```python
from build123d import *

# Parameters (mm, degrees)
F0_W     = 27.4
F0_H     = 2.1
F1_DEPTH = 5
F2_DEPTH = 4
F3_D     = 5
F4_R     = 4.9999


# Not quite as in the source:
# - a fillet or chamfer is up to 0.001 mm smaller than in the source, because OpenCascade refuses the exact size
# - ends of sketch curves that miss each other by under 0.0002 mm in the source are joined
# - a feature names something its author has since deleted; it is built from what else it names


with BuildPart() as f1:
    # F0 (on Top) → F1 (new body)
    with BuildSketch(Plane.XY):
        with BuildLine():
            Line((-35, 2.1762e-06), (-35, -40))
            Line((-35, -40), (-27, -40))
            Line((-27, -40), (-27, -22.2710574513))
            ThreePointArc((-27, -22.2710574513), (-32.9393385518, -11.8321585422), (-35, 2.1762e-06))
        make_face()
        with BuildLine():
            Line((-27, -22.2710574513), (-27, -40))
            Line((-27, -40), (27, -40))
            Line((27, -40), (27, -22.2710574513))
            ThreePointArc((27, -22.2710574513), (0, -35), (-27, -22.2710574513))
        make_face()
        with BuildLine():
            add(Edge.make_bspline(
                [(0, 45), (-20.1986748725, 45), (-35, 20.0504870868), (-35, 2.1762e-06)],
                knots=[0, 0, 0, 0, 57.0087695372, 57.0087695372, 57.0087695372, 57.0087695372], degree=3))
            ThreePointArc((-35, 2.1762e-06), (-28.4666369261, 20.3629708568), (-11.3056830814, 33.1237306181))
            add(Edge.make_bspline(
                [(0, 37), (-0.2833414452, 37.0069688983), (-1.1232932293, 37.0068386903), (-2.7957299856, 36.8864035146), (-4.9942322029, 36.3521195303), (-7.6997383876, 35.2871018647), (-9.7958540485, 34.148638444), (-11.0540635502, 33.3003360386), (-11.3056830814, 33.1237306181)],
                knots=[0, 0, 0, 0, 0.8506820357, 2.5185967411, 5.0181648841, 7.6012051941, 11.2266191262, 12.1476935207, 12.1476935207, 12.1476935207, 12.1476935207], degree=3))
            add(Edge.make_bspline(
                [(0, 37), (0.2833414452, 37.0069688983), (1.1232932293, 37.0068386903), (2.7957299856, 36.8864035146), (4.9942322029, 36.3521195303), (7.6997383876, 35.2871018647), (9.7958540485, 34.148638444), (11.0540635502, 33.3003360386), (11.3056830814, 33.1237306181)],
                knots=[0, 0, 0, 0, 0.8506820357, 2.5185967411, 5.0181648841, 7.6012051941, 11.2266191262, 12.1476935207, 12.1476935207, 12.1476935207, 12.1476935207], degree=3))
            ThreePointArc((11.3056830814, 33.1237306181), (28.4666375592, 20.3629699719), (35, 0))
            add(Edge.make_bspline(
                [(0, 45), (20.1986748725, 45), (35, 20.0504870868), (35, 0)],
                knots=[0, 0, 0, 0, 57.0087695372, 57.0087695372, 57.0087695372, 57.0087695372], degree=3))
        make_face()
        with BuildLine():
            ThreePointArc((-11.3056830814, 33.1237306181), (-28.4666369261, 20.3629708568), (-35, 2.1762e-06))
            ThreePointArc((-35, 2.1762e-06), (-32.9393385518, -11.8321585422), (-27, -22.2710574513))
            Line((-27, -22.2710574513), (-27, 2.1762e-06))
            add(Edge.make_bspline(
                [(-11.3056830814, 33.1237306181), (-12.4097508436, 32.3488132243), (-15.1414824386, 30.0752135158), (-18.8876274503, 25.5283101279), (-22.422035633, 19.604279738), (-25.0662594291, 13.1120426553), (-26.6478130576, 7.1844788974), (-27.0173066601, 2.7756083867), (-27.018694794, 0.6711028041), (-27, 2.1762e-06)],
                knots=[12.1476935207, 12.1476935207, 12.1476935207, 12.1476935207, 16.189226149, 22.7543847852, 29.7183326598, 36.8091409701, 43.7289829573, 48.0262708445, 50.0404462243, 50.0404462243, 50.0404462243, 50.0404462243], degree=3))
        make_face()
        with BuildLine():
            Line((27, -22.2710574513), (27, -40))
            Line((27, -40), (35, -40))
            Line((35, -40), (35, 0))
            ThreePointArc((35, 0), (32.939338184, -11.8321595662), (27, -22.2710574513))
        make_face()
        with BuildLine():
            Line((27, 2.1762e-06), (27, -22.2710574513))
            ThreePointArc((27, -22.2710574513), (32.939338184, -11.8321595662), (35, 0))
            ThreePointArc((35, 0), (28.4666375592, 20.3629699719), (11.3056830814, 33.1237306181))
            add(Edge.make_bspline(
                [(11.3056830814, 33.1237306181), (12.4097508436, 32.3488132243), (15.1414824386, 30.0752135158), (18.8876274503, 25.5283101279), (22.422035633, 19.604279738), (25.0662594291, 13.1120426553), (26.6478130576, 7.1844788974), (27.0173066601, 2.7756083867), (27.018694794, 0.6711028041), (27, 2.1762e-06)],
                knots=[12.1476935207, 12.1476935207, 12.1476935207, 12.1476935207, 16.189226149, 22.7543847852, 29.7183326598, 36.8091409701, 43.7289829573, 48.0262708445, 50.0404462243, 50.0404462243, 50.0404462243, 50.0404462243], degree=3))
        make_face()
        with BuildLine():
            add(Edge.make_bspline(
                [(0, 37), (-0.2833414452, 37.0069688983), (-1.1232932293, 37.0068386903), (-2.7957299856, 36.8864035146), (-4.9942322029, 36.3521195303), (-7.6997383876, 35.2871018647), (-9.7958540485, 34.148638444), (-11.0540635502, 33.3003360386), (-11.3056830814, 33.1237306181)],
                knots=[0, 0, 0, 0, 0.8506820357, 2.5185967411, 5.0181648841, 7.6012051941, 11.2266191262, 12.1476935207, 12.1476935207, 12.1476935207, 12.1476935207], degree=3))
            ThreePointArc((-11.3056830814, 33.1237306181), (0, 35), (11.3056830814, 33.1237306181))
            add(Edge.make_bspline(
                [(0, 37), (0.2833414452, 37.0069688983), (1.1232932293, 37.0068386903), (2.7957299856, 36.8864035146), (4.9942322029, 36.3521195303), (7.6997383876, 35.2871018647), (9.7958540485, 34.148638444), (11.0540635502, 33.3003360386), (11.3056830814, 33.1237306181)],
                knots=[0, 0, 0, 0, 0.8506820357, 2.5185967411, 5.0181648841, 7.6012051941, 11.2266191262, 12.1476935207, 12.1476935207, 12.1476935207, 12.1476935207], degree=3))
        make_face()
        with BuildLine():
            Line((-27, 2.1762e-06), (-27, -22.2710574513))
            ThreePointArc((-27, -22.2710574513), (0, -35), (27, -22.2710574513))
            Line((27, -22.2710574513), (27, 2.1762e-06))
            add(Edge.make_bspline(
                [(11.3056830814, 33.1237306181), (12.4097508436, 32.3488132243), (15.1414824386, 30.0752135158), (18.8876274503, 25.5283101279), (22.422035633, 19.604279738), (25.0662594291, 13.1120426553), (26.6478130576, 7.1844788974), (27.0173066601, 2.7756083867), (27.018694794, 0.6711028041), (27, 2.1762e-06)],
                knots=[12.1476935207, 12.1476935207, 12.1476935207, 12.1476935207, 16.189226149, 22.7543847852, 29.7183326598, 36.8091409701, 43.7289829573, 48.0262708445, 50.0404462243, 50.0404462243, 50.0404462243, 50.0404462243], degree=3))
            ThreePointArc((11.3056830814, 33.1237306181), (0, 35), (-11.3056830814, 33.1237306181))
            add(Edge.make_bspline(
                [(-11.3056830814, 33.1237306181), (-12.4097508436, 32.3488132243), (-15.1414824386, 30.0752135158), (-18.8876274503, 25.5283101279), (-22.422035633, 19.604279738), (-25.0662594291, 13.1120426553), (-26.6478130576, 7.1844788974), (-27.0173066601, 2.7756083867), (-27.018694794, 0.6711028041), (-27, 2.1762e-06)],
                knots=[12.1476935207, 12.1476935207, 12.1476935207, 12.1476935207, 16.189226149, 22.7543847852, 29.7183326598, 36.8091409701, 43.7289829573, 48.0262708445, 50.0404462243, 50.0404462243, 50.0404462243, 50.0404462243], degree=3))
        make_face()
        Polygon((-13.7, -23.2), (-13.7, 0), (-13.7, 2.1), (13.7, 2.1), (13.7, 0), (13.7, -23.2), (13.7, -25.3), (-13.7, -25.3), align=None, mode=Mode.SUBTRACT)
        with Locations((0, 1.05)):
            Rectangle(F0_W, F0_H)
        with Locations((0, -24.25)):
            Rectangle(F0_W, F0_H)
    extrude(amount=F1_DEPTH)

    # F0 (on Top) → F2 (cut)
    with BuildSketch(Plane.XY):
        with Locations((0, 1.05)):
            Rectangle(F0_W, F0_H)
        with Locations((0, -24.25)):
            Rectangle(F0_W, F0_H)
    extrude(amount=F2_DEPTH, mode=Mode.SUBTRACT)

    # F3 (through all)
    with Locations(Plane(origin=(0, 0, 0), x_dir=(1, 0, 0), z_dir=(0, 0, -1))):
        with Locations((0, -37), (-7.7739062126, -35.111513252), (-14.2579257305, -30.4256311694), (-19.3371352018, -24.244884358), (-23.1543015859, -17.2142911543), (-25.7431047524, -9.6447404302), (-26.9552512695, -1.7371048277), (-27, 6.2627700182), (-27, 14.2627700182), (-27, 22.2627700182), (7.7739062126, -35.111513252), (14.2579257305, -30.4256311694), (19.3371352018, -24.244884358), (23.1543015859, -17.2142911543), (25.7431047524, -9.6447404302), (26.9552512695, -1.7371048277), (27, 6.2627700182), (27, 14.2627700182), (27, 22.2627700182), (-27, 30.2627700182), (27, 30.2627700182)):
            Hole(F3_D / 2)

    # F4 (radius 5 in the source; OpenCascade refuses exactly that, so slightly less here)
    f4_edges = [f1.edges().sort_by_distance(p)[0] for p in [
        (-35, -40, 2.5),
        (35, -40, 2.5),
        (-35, -19.999999, 5),
        (0, -40, 5),
    ]]
    fillet(f4_edges, radius=F4_R)


solid = f1.part
```
Check sheet for the modelled part. Datum: model origin and axes. Units: mm. A direction names the side the tool comes from. Coordinates: 2 decimals unless noted, no trailing zeros. Write item = value, one per line. Start each with the question number.
1. Mould release check, pull along Y, two halves, no side actions. Record for faces 3 (the cylindrical face through (20.845, 18.172, 2.535)), 4 (the cylindrical face through (0, -39, 3)), 5 (the cylindrical face through (-27.09, 7.54, 2.53)), 6 (the flat face through (0, 3, 5)): pulls with the +Y half, pulls with the -Y half, needs draft (parallel to the pull), parting line crosses it, or undercut.
2. Thickness scan on probe 1 along Y at (x, z) = (21, 3.95); probe 2 along X at (y, z) = (37, 3.3); probe 3 along Y at (x, z) = (12, 2.5). Record the ranges inside material, lowest first.
3. Tool access check on faces 1 (the cylindrical face through (27.497, 4.178, 2.535)), 2 (the flat face through (0, 1, 4)). Record the directions out of +Z, -Z, +X, -X, +Y, -Y that give a thin tool (end or side, any length) a straight path to the whole face; none if there is none.
4. Sectioned sample at A-A (x = 0). State how many separate pieces and enclosed holes the cut face has, then the cut area to 3 significant figures.
5. Go/stop test with flat-tipped pins: pin 1 (3 mm diameter, centred on x = 5, z = 1, fed in from -Y); pin 2 (1.2 mm diameter, centred on x = 4, z = 1.5, fed in from +Y); pin 3 (3 mm diameter, centred on y = 29.5, z = 0.5, fed in from -X); pin 4 (1.7 mm diameter, centred on x = -1.5, y = 0.5, fed in from -Z). Record where each tip stops, or that it passes through.
The answers:
q1.face_3 = undercut
q1.face_4 = pulls with the -Y half
q1.face_5 = undercut
q1.face_6 = needs draft
q2.probe_1 = -38.07 to 15.95, 18.48 to 22.38, 26.11 to 32.1
q2.probe_2 = -17.06 to -9.41, -6.14 to -2.5, 2.5 to 6.14, 9.41 to 17.06
q2.probe_3 = -39.33 to -25.3, 2.1 to 29.35, 31.5 to 41.18
q3.face_1 = +Z, -Z
q3.face_2 = -Z
q4.separate_pieces = 3
q4.enclosed_holes = 0
q4.area = 256 mm²
q5.pin_1 = -40
q5.pin_2 = 44.62
q5.pin_3 = -26.42
q5.pin_4 = 4
